The model under review builds one solid part; all positions refer to its coordinate system, in mm. Give positions to 0.01 mm unless a question says otherwise; leave off trailing zeros. Loops run counter-clockwise (first coordinate to the right, second up) from the corner with the lowest first, then second, coordinate; pieces in that order, holes last. Notation, with made-up numbers: M -31,22.5 L -23,22.5 A17 cw -23,35.5 Z; hole C -16.5,25.25 d8. An arc over 180 degrees is marked long. Put each result on its own line as item: value. Start each with the question number.
from build123d import *

# Parameters (mm, degrees)
SKETCH1_W                       = 482.6
SKETCH1_H                       = 304.8
BOSS_EXTRUDE1_DEPTH             = 26.416
CUT_EXTRUDE3_DEPTH              = 3.175
SKETCH3_R                       = 6.35
SKETCH3_R_2                     = 2.54
CUT_EXTRUDE2_DEPTH              = 27.416
M10_CLEARANCE_HOLE2_D           = 12
M10_CLEARANCE_HOLE2_CSINK_D     = 12.05
M10_CLEARANCE_HOLE2_CSINK_ANGLE = 90
M10_CLEARANCE_HOLE3_D           = 12
M10_CLEARANCE_HOLE3_CSINK_D     = 12.05
M10_CLEARANCE_HOLE3_CSINK_ANGLE = 90


with BuildPart() as part:
    # Sketch1 → Boss-Extrude1 (new body)
    with BuildSketch(Plane(origin=(0, 0, 0), x_dir=(1, 0, 0), z_dir=(0, 1, 0))):
        Rectangle(SKETCH1_W, SKETCH1_H)
    extrude(amount=BOSS_EXTRUDE1_DEPTH)

    # Sketch2 → Cut-Extrude3 (cut)
    with BuildSketch(Plane(origin=(0, 26.416, 0), x_dir=(1, 0, 0), z_dir=(0, 1, 0))):
        with BuildLine():
            Line((-71.501, 120.142), (-71.501, -120.142))
            ThreePointArc((-71.501, -120.142), (-64.8335, -113.4745), (-58.166, -120.142))
            Line((-58.166, -120.142), (-58.166, 120.142))
            ThreePointArc((-58.166, 120.142), (-64.8335, 113.4745), (-71.501, 120.142))
        make_face()
        with BuildLine():
            ThreePointArc((-58.166, 120.142), (-64.8335, 126.8095), (-71.501, 120.142))
            Line((-71.501, 120.142), (-58.166, 120.142))
        make_face()
        with BuildLine():
            Line((-58.166, 120.142), (-71.501, 120.142))
            ThreePointArc((-71.501, 120.142), (-64.8335, 113.4745), (-58.166, 120.142))
        make_face()
        with BuildLine():
            ThreePointArc((-58.166, -120.142), (-64.8335, -113.4745), (-71.501, -120.142))
            Line((-71.501, -120.142), (-58.166, -120.142))
        make_face()
        with BuildLine():
            Line((-58.166, -120.142), (-71.501, -120.142))
            ThreePointArc((-71.501, -120.142), (-64.8335, -126.8095), (-58.166, -120.142))
        make_face()
        with BuildLine():
            ThreePointArc((58.166, 120.142), (64.8335, 113.4745), (71.501, 120.142))
            Line((71.501, 120.142), (58.166, 120.142))
        make_face()
        with BuildLine():
            Line((58.166, 120.142), (71.501, 120.142))
            ThreePointArc((71.501, 120.142), (64.8335, 126.8095), (58.166, 120.142))
        make_face()
        with BuildLine():
            Line((71.501, -120.142), (71.501, 120.142))
            ThreePointArc((71.501, 120.142), (64.8335, 113.4745), (58.166, 120.142))
            Line((58.166, 120.142), (58.166, -120.142))
            ThreePointArc((58.166, -120.142), (64.8335, -113.4745), (71.501, -120.142))
        make_face()
        with BuildLine():
            ThreePointArc((58.166, -120.142), (64.8335, -126.8095), (71.501, -120.142))
            Line((71.501, -120.142), (58.166, -120.142))
        make_face()
        with BuildLine():
            Line((58.166, -120.142), (71.501, -120.142))
            ThreePointArc((71.501, -120.142), (64.8335, -113.4745), (58.166, -120.142))
        make_face()
    extrude(amount=-CUT_EXTRUDE3_DEPTH, mode=Mode.SUBTRACT)

    # Sketch3 → Cut-Extrude2 (cut, through all)
    with BuildSketch(Plane(origin=(0, 26.416, 0), x_dir=(1, 0, 0), z_dir=(0, 1, 0))):
        with Locations((-211.201, -80.01)):
            Circle(SKETCH3_R)
        with Locations((-211.201, 80.01)):
            Circle(SKETCH3_R)
        with Locations((211.201, -80.01)):
            Circle(SKETCH3_R)
        with Locations((211.201, 80.01)):
            Circle(SKETCH3_R)
        with Locations((-211.201, -127)):
            Circle(SKETCH3_R_2)
        with Locations((-211.201, 127)):
            Circle(SKETCH3_R_2)
        with Locations((211.201, -127)):
            Circle(SKETCH3_R_2)
        with Locations((211.201, 127)):
            Circle(SKETCH3_R_2)
    extrude(amount=-CUT_EXTRUDE2_DEPTH, mode=Mode.SUBTRACT)

    # M10 Clearance Hole2 (through all)
    with Locations(Plane(origin=(0, 26.416, 0), x_dir=(1, 0, 0), z_dir=(0, 1, 0))):
        with Locations((-211.201, -127)):
            CounterSinkHole(M10_CLEARANCE_HOLE2_D / 2, M10_CLEARANCE_HOLE2_CSINK_D / 2, counter_sink_angle=M10_CLEARANCE_HOLE2_CSINK_ANGLE)

    # M10 Clearance Hole3 (through all)
    with Locations(Plane(origin=(0, 26.416, 0), x_dir=(1, 0, 0), z_dir=(0, 1, 0))):
        with Locations((-211.201, 127), (211.201, 127), (211.201, -127)):
            CounterSinkHole(M10_CLEARANCE_HOLE3_D / 2, M10_CLEARANCE_HOLE3_CSINK_D / 2, counter_sink_angle=M10_CLEARANCE_HOLE3_CSINK_ANGLE)


solid = part.part
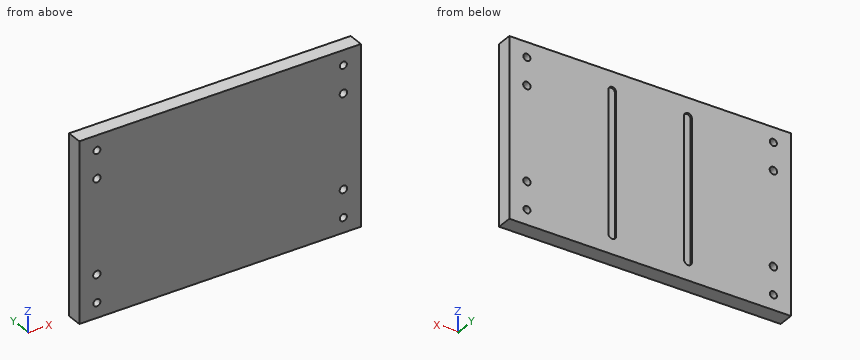
(1) We need section B-B, the plane x = -210. State how many separate pieces and enclosed holes the cut face has, plus the area to 3 significant figures.
(2) We need section A-A, the plane z = 80.01. Write out the cut boundary in (x, y).
(3) Insertion check: pin 1 (7 mm diameter, centred on x = -211.201, z = -127, fed in from +Y); pin 2 (6.5 mm diameter, centred on x = 65.5, z = -32.5, fed in from +Y). Each pin has a flat end and moves straight along its axis. Give the tip position at first contact, or say it passes through.
(4) To check wall thickness, follow L1, parallel to X at y = 16.25, z = -127; L2, parallel to X at y = 8.5, z = 80.01; L3, parallel to Z at x = -213.5, y = 2.5. State the ranges of each line that lie inside material, in increasing order. Write a range as [from, to].
Check sheet entries:
1. separate pieces: 5
1. enclosed holes: 0
1. area: 6,770 mm²
2. outline: M -241.3,0 L -217.55,0 L -217.55,26.42 L -241.3,26.42 Z; M -204.85,0 L 204.85,0 L 204.85,26.42 L 71.5,26.42 L 71.5,23.24 L 58.17,23.24 L 58.17,26.42 L -58.17,26.42 L -58.17,23.24 L -71.5,23.24 L -71.5,26.42 L -204.85,26.42 Z; M 217.55,0 L 241.3,0 L 241.3,26.42 L 217.55,26.42 Z
3. pin 1: passes through
3. pin 2: stops at y = 23.24
4. L1: x = [-241.3, -217.2], [-205.2, 205.2], [217.2, 241.3]
4. L2: x = [-241.3, -217.55], [-204.85, 204.85], [217.55, 241.3]
4. L3: z = [-152.4, -132.54], [-121.46, -85.93], [-74.09, 74.09], [85.93, 121.46], [132.54, 152.4]
